The model under review builds one solid part; all positions refer to its coordinate system, in mm. A direction names the side the tool comes from. Give positions to 0.01 mm unless a question says otherwise; leave off trailing zeros. Write each loop counter-clockwise with the first axis right and the second up, starting at its lowest first coordinate (ties: lowest second). Pieces come first, ordered by that corner, then holes.
from build123d import *

# Parameters (mm, degrees)
BOSS_EXTRUDE1_DEPTH                 = 20
FILLET1_R                           = 10
SKETCH3_R                           = 5.4
CUT_EXTRUDE3_DEPTH                  = 1.23
CUT_EXTRUDE3_DIRECTION_2_REACH      = 81.023
CUT_EXTRUDE3_DIRECTION_2_END_RADIUS = 28.405
SKETCH4_R                           = 3.64
CUT_EXTRUDE4_DEPTH                  = 81.10998653
SKETCH5_R                           = 2.5
CUT_EXTRUDE5_DEPTH                  = 59.869498141


with BuildPart() as part:
    # Sketch2 → Boss-Extrude1 (new body)
    with BuildSketch(Plane.XY):
        with BuildLine():
            Line((-10, -29.770354801), (-10, -32.905))
            Line((-10, -32.905), (10, -32.905))
            Line((10, -32.905), (10, -29.770354801))
            ThreePointArc((10, -29.770354801), (31.318108327, 2.334548309), (5.475658873, 30.923958105))
            Line((5.475658873, 30.923958105), (5.475658873, 41.296910399))
            Line((5.475658873, 41.296910399), (2.475658873, 41.296910399))
            Line((2.475658873, 41.296910399), (2.475658873, 28.296910399))
            ThreePointArc((2.475658873, 28.296910399), (0, -28.405), (-2.475658873, 28.296910399))
            Line((-2.475658873, 28.296910399), (-2.475658873, 41.296910399))
            Line((-2.475658873, 41.296910399), (-5.475658873, 41.296910399))
            Line((-5.475658873, 41.296910399), (-5.475658873, 30.923958105))
            ThreePointArc((-5.475658873, 30.923958105), (-31.318108327, 2.334548309), (-10, -29.770354801))
        make_face()
    extrude(amount=BOSS_EXTRUDE1_DEPTH)

    # Fillet1
    # the kernel refuses this fillet: 10 mm, written as the material it adds along each edge
    with BuildSketch(Plane(origin=(10, -29.770354801, 0), x_dir=(0, -1, 0), z_dir=(0, 0, 1))) as fillet1_piece_1:
        with BuildLine():
            CenterArc((6.874989117, 9.274148337), FILLET1_R, 207.74277492, 40.292580152)
            Line((-1.975474334, 4.619119153), (-2.152483603, 4.526018569))
            ThreePointArc((-2.152483603, 4.526018569), (-1.079113359, 2.270480411), (-0.189589905, -0.063684127))
            Line((-0.189589905, -0.063684127), (0, -0.2))
            ThreePointArc((0, -0.2), (1.567322599, -0.2), (3.05983832, -0.185482967))
            Line((3.05983832, -0.185482967), (3.134645199, 0))
        make_face()
    extrude(amount=20)
    with BuildSketch(Plane(origin=(-10, -29.770354801, 0), x_dir=(0, -1, 0), z_dir=(0, 0, 1))) as fillet1_piece_2:
        with BuildLine():
            CenterArc((6.874989117, -9.274148337), FILLET1_R, 111.964644928, 40.292580152)
            Line((-1.975474334, -4.619119153), (-2.152483603, -4.526018569))
            ThreePointArc((-2.152483603, -4.526018569), (-1.079113359, -2.270480411), (-0.189589905, 0.063684127))
            Line((-0.189589905, 0.063684127), (0, 0.2))
            ThreePointArc((0, 0.2), (1.567322599, 0.2), (3.05983832, 0.185482967))
            Line((3.05983832, 0.185482967), (3.134645199, 0))
        make_face()
    extrude(amount=20)

    # Sketch3 → Cut-Extrude3 (cut)
    with BuildSketch(Plane(origin=(0, -28.405, 0), x_dir=(1, 0, 0), z_dir=(0, 1, 0))):
        with Locations(Location((0, -10, 0), (0, 0, 90))):
            Circle(SKETCH3_R)
    extrude(amount=-CUT_EXTRUDE3_DEPTH, mode=Mode.SUBTRACT)

    # Cut-Extrude3 direction 2: up to this cylinder (the profile starts outside it)
    cut_extrude3_direction_2_end = Plane(origin=(0, 0, 10), z_dir=(0, 0, -1)) * Cylinder(CUT_EXTRUDE3_DIRECTION_2_END_RADIUS, 219.856, mode=Mode.PRIVATE)
    # Sketch3 → Cut-Extrude3 direction 2 (cut, up to the surface)
    with BuildSketch(Plane(origin=(0, -28.405, 0), x_dir=(1, 0, 0), z_dir=(0, 1, 0)), mode=Mode.PRIVATE) as cut_extrude3_direction_2_sk1:
        with Locations(Location((0, -10, 0), (0, 0, 90))):
            Circle(SKETCH3_R)
    cut_extrude3_direction_2_tool1 = extrude(cut_extrude3_direction_2_sk1.sketch, amount=CUT_EXTRUDE3_DIRECTION_2_REACH, mode=Mode.PRIVATE) - cut_extrude3_direction_2_end
    add(cut_extrude3_direction_2_tool1.solids().sort_by_distance((0, -28.405, 10))[0], mode=Mode.SUBTRACT)
    add(cut_extrude3_direction_2_tool1.solids().sort_by_distance((0, -28.405, 10))[1], mode=Mode.SUBTRACT)

    # Sketch4 → Cut-Extrude4 (cut, through all)
    with BuildSketch(Plane(origin=(0, -29.635, 0), x_dir=(1, 0, 0), z_dir=(0, 1, 0))):
        with Locations(Location((0, -10, 0), (0, 0, 180))):
            Circle(SKETCH4_R)
    extrude(amount=-CUT_EXTRUDE4_DEPTH, mode=Mode.SUBTRACT)

    # Sketch5 → Cut-Extrude5 (cut, through all)
    with BuildSketch(Plane.ZY.offset(5.475658873)):
        with Locations(Location((10, 36.110434252, 0), (0, 0, 270))):
            Circle(SKETCH5_R)
    extrude(amount=-CUT_EXTRUDE5_DEPTH, mode=Mode.SUBTRACT)


solid = part.part
1) Consider section D-D, the plane z = 17. Give the boundary of the cut face in (x, y) (3 decimals), then the cut area to 3 significant figures.
2) Insertion check: pin 1 (6.5 mm diameter, centred on y = 36.11, z = 10, fed in from +X); pin 2 (12 mm diameter, centred on x = 10.5, y = 20, fed in from -Z); pin 3 (10 mm diameter, centred on y = -14, z = 8.5, fed in from -X); pin 4 (4 mm diameter, centred on y = 36.11, z = 10, fed in from +X). Each pin has a flat end and moves straight along its axis. Give the tip position at first contact, or say it passes through.
3) Consider section A-A, the plane z = 10. Give the boundary of the cut face in (x, y) (3 decimals).
4) To check wall thickness, follow probe 1 along X at (y, z) = (0, 7.25) (3 decimals); probe 2 along Z at (x, y) = (0, -32); probe 3 along Y at (x, z) = (-22.5, 16). State the ranges of each line that lie inside material, in increasing order.
5) Consider section C-C, the plane x = 9. Give the boundary of the cut face in (y, z) (1 decimal).
6) Tool access review of faces 5 (the flat face through (-2.476, 33, 10)), 6 (the flat face through (0, -32.905, 5)), 7 (the flat face through (5.476, 34.9, 7.6)), 8 (the flat face through (-5.476, 37.3, 7.6)), 9 (the cylindrical face through (-1.68, -31.25, 6.77)): name each direction out of +Z, -Z, +X, -X, +Y, -Y from which nothing blocks a thin tool from reaching the whole face with its end or side.
7) The part is to be moulded in two halves that separate along Z. For faces 1 (the cylindrical face through (11.89, -29.9, 9.86)), 2 (the flat face through (12, -26, 20)), 3 (the flat face through (1, -29.635, 6)), 4 (the flat face through (12, -26, 0)), say which applies: +Z half, -Z half, draft (parallel to the pull), parting line (faces both ways), or undercut.
8) Consider section B-B, the plane y = 0. Give the boundary of the cut face in (x, z) (3 decimals).
Answer block:
1. outline: (-14.619, -27.795) arc R10 cw to (-10, -32.905) - (10, -32.905) arc R10 cw to (14.619, -27.795) arc R31.405 ccw to (5.476, 30.924) - (5.476, 41.297) - (2.476, 41.297) - (2.476, 28.297) arc R28.405 cw (long way) to (-2.476, 28.297) - (-2.476, 41.297) - (-5.476, 41.297) - (-5.476, 30.924) arc R31.405 ccw to start
1. area: 659 mm2
2. pin 1: stops at x = 5.48
2. pin 2: stops at z = 0
2. pin 3: stops at x = -30.09
2. pin 4: passes through
3. outline: (-14.619, -27.795) arc R10 cw to (-10, -32.905) - (-3.64, -32.905) - (-3.64, -29.635) - (-5.4, -29.635) - (-5.4, -27.887) arc R28.405 cw to (-2.476, 28.297) - (-2.476, 33.61) - (-5.476, 33.61) - (-5.476, 30.924) arc R31.405 ccw to start; (-5.476, 38.61) - (-2.476, 38.61) - (-2.476, 41.297) - (-5.476, 41.297) - close; (2.476, 28.297) arc R28.405 cw to (5.4, -27.887) - (5.4, -29.635) - (3.64, -29.635) - (3.64, -32.905) - (10, -32.905) arc R10 cw to (14.619, -27.795) arc R31.405 ccw to (5.476, 30.924) - (5.476, 33.61) - (2.476, 33.61) - close; (2.476, 38.61) - (5.476, 38.61) - (5.476, 41.297) - (2.476, 41.297) - close
4. probe 1: x = -31.405 to -28.405, 28.405 to 31.405
4. probe 2: z = 0 to 6.36, 13.64 to 20
4. probe 3: y = -21.91 to -17.34, 17.34 to 21.91
5. outline: (-32.9, 0) - (-26.9, 0) - (-26.9, 20) - (-32.9, 20) - close; (26.9, 0) - (30.1, 0) - (30.1, 20) - (26.9, 20) - close
6. face 5: +Z, -Z, +Y
6. face 6: +Z, -Z, +X, -X, -Y
6. face 7: +Z, -Z, +X, +Y
6. face 8: +Z, -Z, -X, +Y
6. face 9: -Y
7. face 1: draft
7. face 2: +Z half
7. face 3: undercut
7. face 4: -Z half
8. outline: (-31.405, 0) - (-28.405, 0) - (-28.405, 20) - (-31.405, 20) - close; (28.405, 0) - (31.405, 0) - (31.405, 20) - (28.405, 20) - close
